The drawing under review shows one solid part. Ordinate dimensions are in mm from its lowest x, y, z. A direction names the side the tool comes from. Coordinates: 2 decimals unless noted, no trailing zeros. Loops run counter-clockwise (first coordinate to the right, second up) from the corner with the lowest first, then second, coordinate; pieces in that order, holes last. Notation, with made-up numbers: (88.25, 30) - (147.25, 30) arc R14 cw to (147.25, 41) - close; hole circle Ø1 at (85.25, 64.5). An arc over 180 degrees is marked (long way). Answer as a JSON object with one key per item and string values. Group by question number.
Item 1: We need section C-C (x = 26). Give the boundary of the cut face in (y, z).
Item 2: Tool access review of the marked faces 4 and 5: name each direction out of +Z, -Z, +X, -X, +Y, -Y from which nothing blocks a thin tool from reaching the whole face with its end or side.
Item 3: We need section B-B (z = 40). Give the boundary of the cut face in (x, y).
Item 4: We need section A-A (y = 40). Give the boundary of the cut face in (x, z), then the cut area to 3 significant figures.
Item 5: To check wall thickness, follow line 1 (Y direction, x = 102, z = 41); line 2 (Y direction, x = 98.5, z = 43) (1 decimal); line 3 (X direction, y = 40, z = 34). State the ranges of each line that lie inside material, in increasing order.
Item 6: Clearance check with flat-ended pins moving along their axes: pin 1 (1.5 mm diameter, centred on x = 23.5, y = 58.5, fed in from +Z) (1 decimal); pin 2 (10 mm diameter, centred on x = 103, z = 44, fed in from +Y); pin 3 (11 mm diameter, centred on x = 102, y = 40, fed in from -Z); pin 4 (10 mm diameter, centred on x = 43, y = 39.5, fed in from +Z). State where each tip first meets the part, or that it passes through.
Item 7: We need section D-D (x = 102). Give the boundary of the cut face in (y, z).
Item 8: Mouldability with a two-part tool opening along Y and no side actions: class the marked faces 1, 2 and 3 as released by +Y, released by -Y, zero draft, split by the parting line, or undercut.
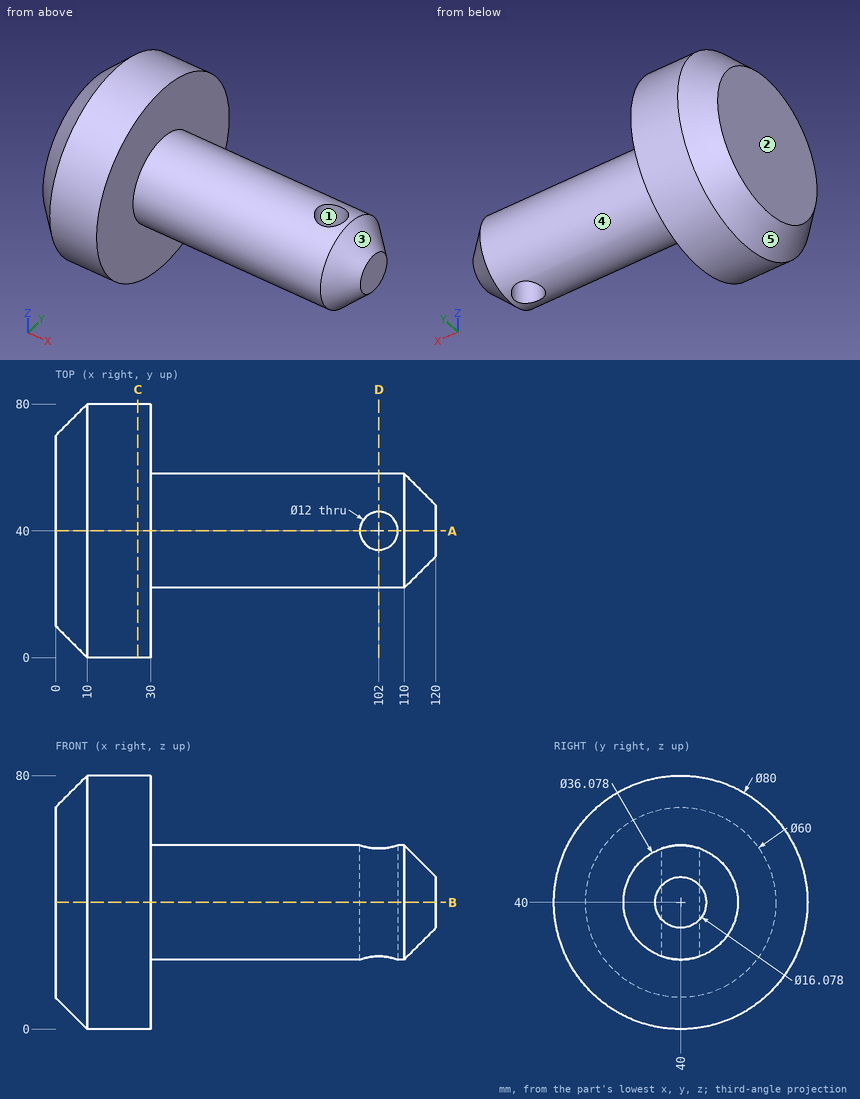
Check sheet entries:
{
 "1": {"outline": "circle Ø80 at (40, 40)"},
 "2": {"face 4": "+X", "face 5": "-X"},
 "3": {"outline": "(0, 10) - (10, 0) - (30, 0) - (30, 21.96) - (110, 21.96) - (120, 31.96) - (120, 48.04) - (110, 58.04) - (30, 58.04) - (30, 80) - (10, 80) - (0, 70) - close; hole circle Ø12 at (102, 40)"},
 "4": {"outline": "(0, 10) - (10, 0) - (30, 0) - (30, 21.96) - (96, 21.96) - (96, 58.04) - (30, 58.04) - (30, 80) - (10, 80) - (0, 70) - close; (108, 21.96) - (110, 21.96) - (120, 31.96) - (120, 48.04) - (110, 58.04) - (108, 58.04) - close", "area": "5,010 mm2"},
 "5": {"line 1": "y = 21.99 to 34, 46 to 58.01", "line 2": "y = 22.2 to 35.1, 44.9 to 57.8", "line 3": "x = 0 to 96, 108 to 120"},
 "6": {"pin 1": "stops at z = 75.8", "pin 2": "stops at y = 58.04", "pin 3": "passes through", "pin 4": "stops at z = 58.04"},
 "7": {"outline": "(34, 22.99) - (34, 57.01) arc R18.04 ccw to start; (46, 22.99) arc R18.04 ccw to (46, 57.01) - close"},
 "8": {"face 1": "undercut", "face 2": "zero draft", "face 3": "split by the parting line"}
}
